```python
from build123d import *

# Parameters (mm, degrees)
SKETCH1_W           = 23
SKETCH1_H           = 12.1
BOSS_EXTRUDE1_DEPTH = 18.4
SKETCH2_W           = 0.8
SKETCH2_H           = 6.3
BOSS_EXTRUDE2_DEPTH = 9.5
SKETCH3_W           = 31.8
SKETCH3_H           = 16.5
BOSS_EXTRUDE3_DEPTH = 2.1
CHAMFER1_SIZE       = 1.5
SKETCH4_W           = 1
SKETCH4_H           = 5
BOSS_EXTRUDE4_DEPTH = 2.1
CUT_EXTRUDE1_DEPTH  = 1
SKETCH7_W           = 21
SKETCH7_H           = 9.5
BOSS_EXTRUDE5_DEPTH = 6
CUT_EXTRUDE3_DEPTH  = 9.5


with BuildPart() as part:
    # Sketch1 → Boss-Extrude1 (new body)
    with BuildSketch(Plane(origin=(0, 0, 0), x_dir=(1, 0, 0), z_dir=(0, 1, 0))):
        with Locations((11.5, 6.05)):
            Rectangle(SKETCH1_W, SKETCH1_H)
    extrude(amount=BOSS_EXTRUDE1_DEPTH)

    # Sketch2 → Boss-Extrude2 (add)
    with BuildSketch(Plane.XZ):
        with Locations((2, -6.05)):
            Rectangle(SKETCH2_W, SKETCH2_H)
        with Locations((11.5, -6.05)):
            Rectangle(SKETCH2_W, SKETCH2_H)
    extrude(amount=BOSS_EXTRUDE2_DEPTH)

    # Sketch3 → Boss-Extrude3 (add)
    with BuildSketch(Plane(origin=(0, 18.4, 0), x_dir=(1, 0, 0), z_dir=(0, 1, 0))):
        with Locations((11.5, 6.05)):
            Rectangle(SKETCH3_W, SKETCH3_H)
    extrude(amount=BOSS_EXTRUDE3_DEPTH)

    # Chamfer1
    chamfer1_edges = [part.edges().sort_by_distance(p)[0] for p in [
        (-4.4, 20.5, -6.05),
        (11.5, 20.5, 2.2),
        (27.4, 20.5, -6.05),
        (11.5, 20.5, -14.3),
    ]]
    chamfer(chamfer1_edges, length=CHAMFER1_SIZE)

    # Sketch4 → Boss-Extrude4 (add)
    with BuildSketch(Plane.ZY):
        with Locations((-6.05, 15.9)):
            Rectangle(SKETCH4_W, SKETCH4_H)
    boss_extrude4 = extrude(amount=BOSS_EXTRUDE4_DEPTH)

    # Sketch5 → Cut-Extrude1 (cut)
    with BuildSketch(Plane.XY.offset(-5.55)):
        with BuildLine():
            ThreePointArc((-0.312308302, 13.4), (-1.535088668, 13.964911332), (-2.1, 15.187691698))
            Line((-2.1, 15.187691698), (-2.1, 13.4))
            Line((-2.1, 13.4), (-0.312308302, 13.4))
        make_face()
    cut_extrude1 = extrude(amount=-CUT_EXTRUDE1_DEPTH, mode=Mode.SUBTRACT)

    # Mirror2: Boss-Extrude4 across plane
    add(boss_extrude4.mirror(Plane.ZY.offset(-11.5)))

    # Mirror3: Cut-Extrude1 across plane
    add(cut_extrude1.mirror(Plane.ZY.offset(-11.5)), mode=Mode.SUBTRACT)

    # Sketch7 → Boss-Extrude5 (add)
    with BuildSketch(Plane(origin=(0, 20.5, 0), x_dir=(1, 0, 0), z_dir=(0, 1, 0))):
        with Locations((11.5, 6.05)):
            Rectangle(SKETCH7_W, SKETCH7_H)
    extrude(amount=BOSS_EXTRUDE5_DEPTH)

    # Sketch8 → Cut-Extrude3 (cut)
    with BuildSketch(Plane.XY.offset(-1.3)):
        with BuildLine():
            ThreePointArc((1, 21.544517728), (2.080144811, 24.495369861), (4.5, 26.5))
            Line((4.5, 26.5), (1, 26.5))
            Line((1, 26.5), (1, 21.544517728))
        make_face()
        with BuildLine():
            Line((1, 20.5), (1, 21.544517728))
            ThreePointArc((1, 21.544517728), (0.977304154, 21.022258864), (1, 20.5))
        make_face()
        with BuildLine():
            Line((22, 26.5), (4.5, 26.5))
            ThreePointArc((4.5, 26.5), (12.74453051, 22.025713988), (22, 20.5))
            Line((22, 20.5), (22, 26.5))
        make_face()
    extrude(amount=-CUT_EXTRUDE3_DEPTH, mode=Mode.SUBTRACT)


solid = part.part
```
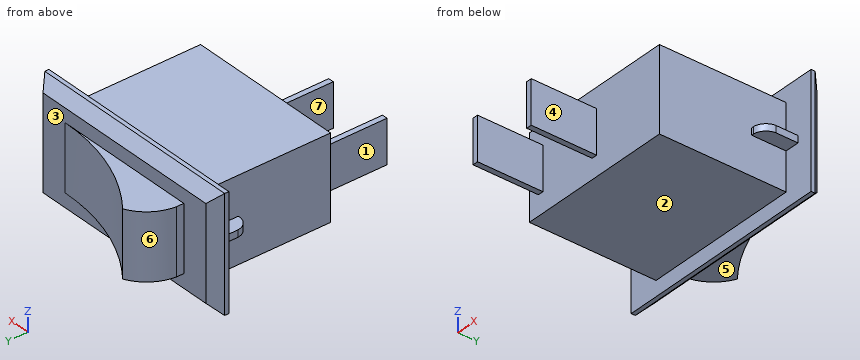
Model file for the job. Use its own axes, mm. Face numbers are marked on the shaded views. A direction names the side the tool comes from. Give positions to 0.01 mm unless a question says otherwise; leave off trailing zeros. Loops run counter-clockwise (first coordinate to the right, second up) from the corner with the lowest first, then second, coordinate; pieces in that order, holes last. Notation, with made-up numbers: (31.25, -36.75) - (43.25, -36.75) arc R17 ccw to (43.25, -24.75) - close; hole circle Ø2 at (-0.75, 64.5). An arc over 180 degrees is marked (long way). One line per item, written item: value. Start each with the question number.
1. Which spindle directions (+Z, -Z, +X, -X, +Y, -Y) get a long thin tool onto all of the face, cutting with end or side? Do the marked faces 1, 2, 3 and 4. Say none if no direction does.
2. Pin check, flat tips, straight feed: pin 1 (7 mm diameter, centred on y = -5, z = -6, fed in from -X); pin 2 (1.1 mm diameter, centred on x = 24.5, y = 15, fed in from +Z); pin 3 (3 mm diameter, centred on x = 7, y = 24.5, fed in from +Z). Stop position of each tip, or through.
3. Probe L1, parallel to Y at x = 21, z = 0.25; L2, parallel to X at y = 8, z = -8.25; L3, parallel to Z at x = 5.5, y = 18. List the from-to ranges inside material, lowest first. Write a range as from..to.
4. Slice it at A-A (y = -4.5). List the corners of the cut face in (x, z), plus the area to 3 significant figures.
5. Pull direction X, two halves, no side cores. Call the marked faces 5, 6 and 7: pulls with the +X half, pulls with the -X half, needs draft (parallel to the pull), parting line crosses it, or undercut.
6. Slice it at B-B (z = -10). List the corners of the cut face in (x, y).
7. Slice it at D-D (z = -7.25). List the corners of the cut face in (x, y), plus the area to 3 significant figures.
Solution:
1. face 1: +Z, -Z, -X, -Y
1. face 2: -Z, +X, -X, -Y
1. face 3: +Y
1. face 4: +Z, -Z, +X, -Y
2. pin 1: stops at x = 1.6
2. pin 2: stops at z = -5.55
2. pin 3: stops at z = -1.3
3. L1: y = 18.4..20.5
3. L2: x = 0..23
3. L3: z = -12.1..0
4. outline: (1.6, -9.2) - (2.4, -9.2) - (2.4, -2.9) - (1.6, -2.9) - close; (11.1, -9.2) - (11.9, -9.2) - (11.9, -2.9) - (11.1, -2.9) - close
4. area: 10.1 mm^2
5. face 5: needs draft
5. face 6: pulls with the -X half
5. face 7: undercut
6. outline: (-4.4, 18.4) - (0, 18.4) - (0, 0) - (23, 0) - (23, 18.4) - (27.4, 18.4) - (27.4, 19) - (25.9, 20.5) - (22, 20.5) arc R28.23 cw to (4.5, 26.5) arc R6.02 ccw to (1, 21.54) - (1, 20.5) - (-2.9, 20.5) - (-4.4, 19) - close
7. outline: (-4.4, 18.4) - (0, 18.4) - (0, 0) - (1.6, 0) - (1.6, -9.5) - (2.4, -9.5) - (2.4, 0) - (11.1, 0) - (11.1, -9.5) - (11.9, -9.5) - (11.9, 0) - (23, 0) - (23, 18.4) - (27.4, 18.4) - (27.4, 19) - (25.9, 20.5) - (22, 20.5) arc R28.23 cw to (4.5, 26.5) arc R6.02 ccw to (1, 21.54) - (1, 20.5) - (-2.9, 20.5) - (-4.4, 19) - close
7. area: 552 mm^2
